Autodesk Inventor part; units mm, degrees
ref_plane "YZ Plane" through (0, 0, 0) normal (1, 0, 0) x (0, 1, 0)
ref_plane "XZ Plane" through (0, 0, 0) normal (0, 1, 0) x (-1, 0, 0)
ref_plane "XY Plane" through (0, 0, 0) normal (0, 0, 1) x (1, 0, 0)
sketch "Sketch1" plane through (0, 0, 0) normal (0, 0, 1) x (1, 0, 0)
  line L0 (-12.7, -12.7) -> (12.7, -12.7)
  line L1 (12.7, -12.7) -> (12.7, 12.7)
  line L2 (12.7, 12.7) -> (-12.7, 12.7)
  line L3 (-12.7, 12.7) -> (-12.7, -12.7)
  line L4 (-12.7, -12.7) -> (12.7, 12.7) construction
  line L5 (12.7, -12.7) -> (-12.7, 12.7) construction
  line L6 (-11.1125, 11.1125) -> (11.1125, 11.1125)
  line L7 (11.1125, 11.1125) -> (11.1125, -11.1125)
  line L8 (11.1125, -11.1125) -> (-11.1125, -11.1125)
  line L9 (-11.1125, -11.1125) -> (-11.1125, 11.1125)
  point P0 (0, 0)
  dimension "width" = 25.4
  dimension "height" = 25.4
  dimension "thickness" = 1.5875
extrude "Extrusion1" add sketch "Sketch1" along normal mid plane 281.1138
sketch "Sketch2" plane through (12.7, -12.7, 140.5569) normal (1, 0, 0) x (0, 0, -1)
  line L0 (281.1138, 25.4) -> (281.1138, 0) construction
  line L1 (281.1138, 0) -> (0, 0) construction
  line L2 (0, 0) -> (0, 25.4) construction
  line L3 (0, 25.4) -> (281.1138, 25.4) construction
  point P0 (140.5569, 12.7)
  point P1 (12.7, 12.7)
  point P2 (38.1, 12.7)
  point P3 (0, 12.7)
  dimension "d5" = 25.4
  dimension "d6" = 12.7
hole "Hole1" at (12.7, 0, 127.8569) at (12.7, 0, 102.4569) direction (-1, 0, 0) diameter 5.1054 end through all
sketch "Sketch3" plane through (12.7, -12.7, 140.5569) normal (1, 0, 0) x (0, 0, -1)
  circle A0 centre (12.7, 12.7) radius 2.5527 construction
  circle A1 centre (38.1, 12.7) radius 2.5527 construction
  line L0 (281.1138, 25.4) -> (0, 25.4) construction
  line L1 (0, 0) -> (0, 25.4) construction
  line L2 (281.1138, 0) -> (0, 0) construction
  line L3 (281.1138, 25.4) -> (281.1138, 0) construction
  line L4 (281.1138, 25.4) -> (0, 25.4) construction
  line L5 (281.1138, 25.4) -> (281.1138, 0) construction
  line L6 (274.3611, 0) -> (281.1138, 0)
  line L7 (281.1138, 0) -> (281.1138, 12.7)
  line L8 (281.1138, 12.7) -> (274.3611, 0)
  point P0 (140.5569, 12.7)
  dimension "d14" = 28
extrude "Extrusion2" cut sketch "Sketch3" against normal through all
sketch "Sketch4" plane through (-12.7, -12.7, 140.5569) normal (-1, 0, 0) x (0, 0, 1)
  line L0 (-281.1138, 12.7) -> (-281.1138, 25.4) construction
  line L1 (-281.1138, 25.4) -> (0, 25.4) construction
  point P0 (-140.5569, 12.7)
  point P1 (-251.4637, 12.6978)
  point P2 (-200.6637, 12.6978)
  point P3 (-149.8637, 12.6978)
  point P4 (-281.1138, 19.05)
  dimension "d19" = 50.8
  dimension "d20" = 50.8
  dimension "d21" = 29.6501
  dimension "d22" = 12.7022
hole "Hole2" at (-12.7, -0.0022, -110.9068) at (-12.7, -0.0022, -60.1068) at (-12.7, -0.0022, -9.3068) direction (1, 0, 0) diameter 5.1054 end through all
properties part number "CL4-007" material "Aluminum 6061"
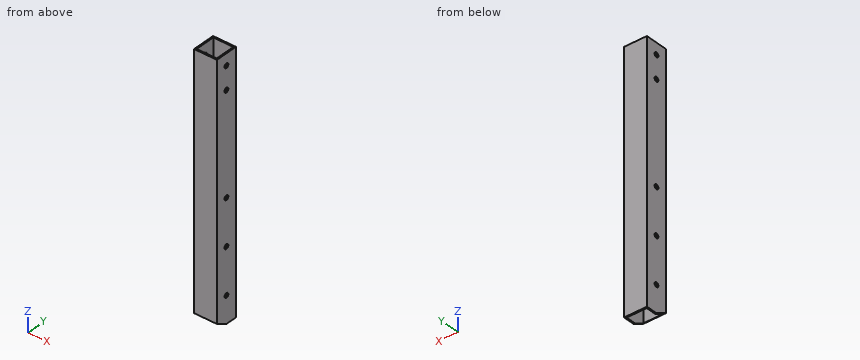
Source: CAD feature listing. Evaluate the final solid. Frame: model axes, mm. Give positions to 0.01 mm unless a question says otherwise; leave off trailing zeros. Loops run counter-clockwise (first coordinate to the right, second up) from the corner with the lowest first, then second, coordinate; pieces in that order, holes last. Notation, with made-up numbers: (-32, -38.75) -> (-21, -38.75) arc R13 cw to (-21, -24.75) -> close; hole circle Ø8 at (18, -35). An arc over 180 degrees is marked (long way). Use a Markdown table: item, result. Add a question column.
1) Line query: line 1 along Z through (x, y) = (11.6, 0); line 2 along Y through (x, z) = (10.5, 105). Output: solid intervals per line, ascending. Write a range as [from, to].
2) Section query A-A, the plane x = 4.25. Return the cut outline in (y, z), then the cut area to 3 significant figures.
3) Section query C-C, the plane y = 6. Return the cut outline in (x, z), then the cut area to 3 significant figures.
4) Section query B-B, the plane z = -51. Return the cut outline in (x, y).
Numbers:
| question | item | result |
|---|---|---|
| 1 | line 1 | z = [-140.56, -113.46], [-108.35, -62.66], [-57.55, -11.86], [-6.75, 99.9], [105.01, 125.3], [130.41, 140.56] |
| 1 | line 2 | y = [-12.7, -11.11], [11.11, 12.7] |
| 2 | outline | (-12.7, -133.8) -> (-11.11, -134.65) -> (-11.11, 140.56) -> (-12.7, 140.56) -> close; (11.11, -140.56) -> (12.7, -140.56) -> (12.7, 140.56) -> (11.11, 140.56) -> close |
| 2 | area | 882 mm2 |
| 3 | outline | (-12.7, -140.56) -> (-11.11, -140.56) -> (-11.11, 140.56) -> (-12.7, 140.56) -> close; (11.11, -140.56) -> (12.7, -140.56) -> (12.7, 140.56) -> (11.11, 140.56) -> close |
| 3 | area | 893 mm2 |
| 4 | outline | (-12.7, -12.7) -> (12.7, -12.7) -> (12.7, 12.7) -> (-12.7, 12.7) -> close; hole (-11.11, -11.11) -> (11.11, -11.11) -> (11.11, 11.11) -> (-11.11, 11.11) -> close |
